Check sheet for the modelled part. Datum: model origin and axes. Units: mm. A direction names the side the tool comes from. Round coordinates to 2 decimals unless told otherwise and drop trailing zeros. Loops run counter-clockwise (first coordinate to the right, second up) from the corner with the lowest first, then second, coordinate; pieces in that order, holes last. Notation, with made-up numbers: (70, 30) - (92, 30) arc R24 ccw to (92, 46) - close; hole circle Ø3 at (54, 31.5). An arc over 180 degrees is marked (long way). Return JSON: item names as keys, results as strings.
from build123d import *

# Parameters (mm, degrees)
SKETCH002_R  = 65
PAD_DEPTH    = 4
POCKET_DEPTH = 20
CHAMFER_SIZE = 7


with BuildPart() as body001:
    # Sketch002 → Pad (new body)
    with BuildSketch(Plane.XY):
        Circle(SKETCH002_R)
    extrude(amount=PAD_DEPTH)


with BuildPart() as body:
    # Sketch → Revolution (revolve)
    with BuildSketch(Plane.XZ):
        Polygon((0, 0), (0, 15), (3.75, 15), (3.75, 3), (56.757359, 3), (58.757359, 1), (61.242641, 1), (63.242641, 3), (96.585786, 3), (98, 4.414214), (98, 20), (100, 20), (100, 0), align=None)
    revolve(axis=Axis((0, 0, 0), (0, 0, 1)))

    # Sketch001 (on DatumPlane) → Pocket (cut)
    with BuildSketch(Plane(origin=(0, 0, 4), x_dir=(-1, 0, 0), z_dir=(0, 0, 1))):
        with BuildLine():
            ThreePointArc((-60, -103.923048), (0, -120), (60, -103.923048))
            Line((32.5, -56.291651), (60, -103.923048))
            ThreePointArc((-32.5, -56.291651), (0, -65), (32.5, -56.291651))
            Line((-32.5, -56.291651), (-60, -103.923048))
        make_face()
    extrude(amount=POCKET_DEPTH, mode=Mode.SUBTRACT)

    # Chamfer
    chamfer_edges = [body.edges().sort_by_distance(p)[0] for p in [
        (-49.396447, 85.557155, 4),
        (49.396447, 85.557155, 4),
    ]]
    chamfer(chamfer_edges, length=CHAMFER_SIZE)

    # Boolean: intersect Body001
    add(body001.part, mode=Mode.INTERSECT)


solid = body.part
Q1. Scan lines: probe 1 along Y at (x, z) = (30, 2.65); probe 2 along Y at (x, z) = (-25, 1.2); probe 3 along X at (y, z) = (-26, 1.75). Record each from-to range of solid material in increasing order. Write a range as [from, to].
Answer key:
{"probe 1": "y = [-57.66, -55.28], [-48.59, 48.59], [55.28, 57.66]", "probe 2": "y = [-60, -56.13], [-52.95, 52.95], [56.13, 60]", "probe 3": "x = [-59.57, -56.28], [-51.85, 51.85], [56.28, 59.57]"}
Q2. Draft check along X on faces 1 (the face through (-12.331, -55.53, 2.875)), 2 (the face through (-14, -62, 3)), 3 (the face through (62, 19.52, 1.48)). Enter one of: released by +X, released by -X, zero draft, split by the parting line, or undercut.
Answer key:
{"face 1": "undercut", "face 2": "zero draft", "face 3": "split by the parting line"}
Q3. Sectioned sample at A-A (x = 0). Enter the section's corners in (y, z), plus the area to 3 significant figures.
Answer key:
{"outline": "(-65, 0) - (65, 0) - (65, 3) - (63.24, 3) - (61.24, 1) - (58.76, 1) - (56.76, 3) - (3.75, 3) - (3.75, 4) - (-3.75, 4) - (-3.75, 3) - (-56.76, 3) - (-58.76, 1) - (-61.24, 1) - (-63.24, 3) - (-65, 3) - close", "area": "380 mm²"}
Q4. Tool access check on faces 4 (the face through (0, 0, 4)), 5 (the face through (23, 55, 1)). Record the directions out of +Z, -Z, +X, -X, +Y, -Y that give a thin tool (end or side, any length) a straight path to the whole face; none if there is none.
Answer key:
{"face 4": "+Z, +X, -X, +Y, -Y", "face 5": "+Z"}
Q5. Depth check by flat-ended pin: P1, Ø1, axis at y = 10.5, z = 1.5, coming from the -X side; P2, Ø8, axis at x = 15, y = 50, coming from the +Z side. Enter the tip coordinate at first touch or a pass-through.
Answer key:
{"P1": "stops at x = -64.23", "P2": "stops at z = 3"}
